Here's the drawing with two shaded views (mm, measured from the low corner). I have some questions. A direction names the side the tool comes from. Give positions to 0.01 mm unless a question says otherwise; leave off trailing zeros. Write each loop counter-clockwise with the first axis right and the second up, starting at its lowest first coordinate (ties: lowest second). Pieces come first, ordered by that corner, then holes. Notation, with made-up numbers: M -4.75,-20 L 34.25,-20 A38 ccw 34.25,19 Z; hole C -25.5,-9 d9. An arc over 180 degrees is marked long. Answer as CSV lines item,"result". Start each with the question number.
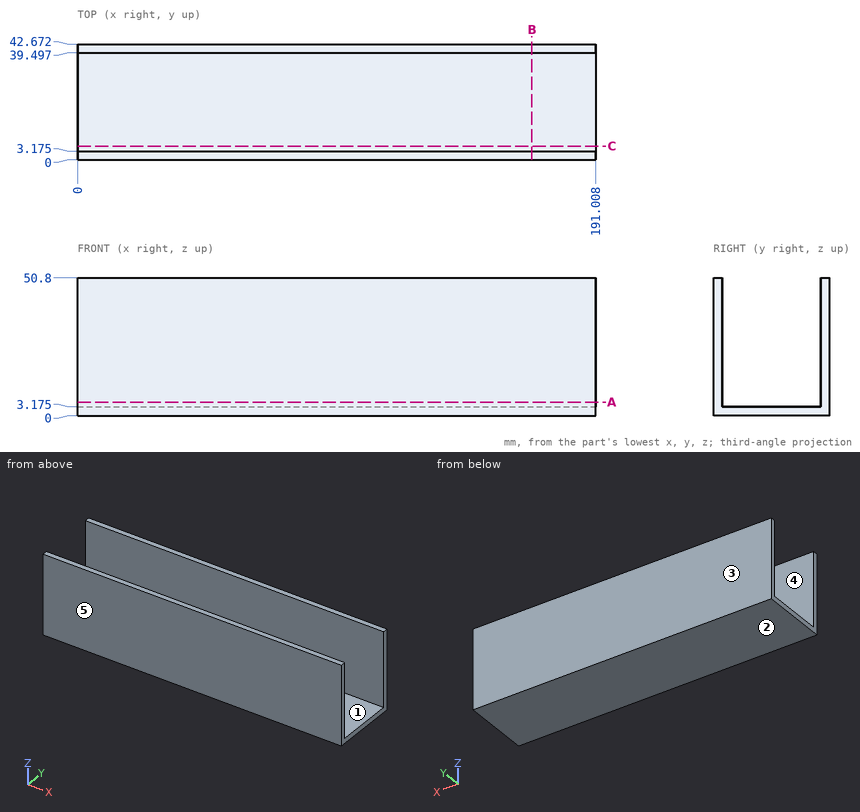
1. Will these pins go through, and if not, where does the flat tip stop? P1, Ø3, axis at x = 53.5, z = 32.5, coming from the -Y side; P2, Ø10, axis at x = 134, y = 31, coming from the +Z side (3 decimals).
2. Imagine slicing it at A-A, the plane z = 5. Please give me the cut outline in (x, y) (3 decimals).
3. Imagine slicing it at C-C, the plane y = 5. Please give me the cut outline in (x, z) (3 decimals), plus the area to 3 significant figures.
4. Imagine slicing it at B-B, the plane x = 167.5. Please give me the cut outline in (y, z) (3 decimals).
5. Thinking about a two-plate mould opening in Y: for the marked faces 1, 2 and 3, which applies, pulls with the +Y half, pulls with the -Y half, needs draft (parallel to the pull), parting line crosses it, or undercut?
6. Please list where these lines run through material, in increasing order: line 1 (Y direction, x = 55, z = 17.5) (3 decimals); line 2 (Z direction, x = 152, y = 20) (3 decimals).
7. On a 3-axis mill with a long thin cutter (end or side, diameter ignored), from which of +Z, -Z, +X, -X, +Y, -Y can I reach the whole of each face in a straight line? I mean the marked faces 4 and 5. Say none if no direction works.
Solutions:
1,P1,"y = 0"
1,P2,"z = 3.175"
2,outline,"M 0,0 L 191.008,0 L 191.008,3.175 L 0,3.175 Z; M 0,39.497 L 191.008,39.497 L 191.008,42.672 L 0,42.672 Z"
3,outline,"M 0,0 L 191.008,0 L 191.008,3.175 L 0,3.175 Z"
3,area,"606 mm²"
4,outline,"M 0,0 L 42.672,0 L 42.672,50.8 L 39.497,50.8 L 39.497,3.175 L 3.175,3.175 L 3.175,50.8 L 0,50.8 Z"
5,face 1,"undercut"
5,face 2,"needs draft"
5,face 3,"pulls with the +Y half"
6,line 1,"0 to 3.175, 39.497 to 42.672"
6,line 2,"0 to 3.175"
7,face 4,"+Z, +X, -X"
7,face 5,"+Z, -Z, +X, -X, -Y"
